from build123d import *

# Parameters (mm, degrees)
F1_DEPTH = 1220
F2_T     = -4


with BuildPart() as f1:
    # F0 (on Right) → F1 (new body)
    with BuildSketch(Plane.YZ):
        with BuildLine():
            Line((0, 40), (0, 0))
            Line((0, 0), (100, 0))
            Line((100, 0), (100, 40))
            ThreePointArc((100, 40), (97.071068, 47.071068), (90, 50))
            Line((90, 50), (10, 50))
            ThreePointArc((10, 50), (2.928932, 47.071068), (0, 40))
        make_face()
    extrude(amount=F1_DEPTH)

    # F2
    f2_openings = [f1.faces().sort_by_distance(p)[0] for p in [
        (610, 50, 0),
        (1220, 50, 24.80288),
        (0, 50, 24.80288),
    ]]
    offset(amount=F2_T, openings=f2_openings)


solid = f1.part
Design review of the part built by this model. Coordinates are the model's own, in mm. A direction names the side the tool comes from. Give positions to 0.01 mm unless a question says otherwise; leave off trailing zeros. Write each loop counter-clockwise with the first axis right and the second up, starting at its lowest first coordinate (ties: lowest second). Pieces come first, ordered by that corner, then holes. Notation, with made-up numbers: M -36,88 L -9,88 A17 cw -9,119 Z; hole C 60.25,41.5 d4. An arc over 180 degrees is marked long. Return JSON: item names as keys, results as strings. Group by question number.
Item 1: Tool access review of faces 4 (the flat face through (601, 51, 46)), 5 (the flat face through (601, 100, 20)): name each direction out of +Z, -Z, +X, -X, +Y, -Y from which nothing blocks a thin tool from reaching the whole face with its end or side.
Item 2: Wall thickness on line 1 along Y through (x, z) = (276, 8); line 2 along Z through (x, y) = (277, 67); line 3 along Z through (x, y) = (221.5, 8): over which ranges is each line inside the solid? List them lowest first.
Item 3: Take a section at C-C (y = 77.5). Give the boundary of the cut face in (x, z), plus the area to 3 significant figures.
Item 4: Take a section at A-A (z = 17). Give the boundary of the cut face in (x, y).
Item 5: Clearance check with a flat-ended pin moving along its axis: pin 1 Ø2 at (x, y) = (367.5, 22.5) entering from -Z. State where the tip first meets the part, or that it passes through.
Item 6: The part is to be moulded in two halves that separate along Y. For faces 1 (the flat face through (601, 0, 20)), 2 (the flat face through (601, 4, 20)), 3 (the flat face through (1220, 50, 47)), say which applies: pulls with the +Y half, pulls with the -Y half, needs draft (parallel to the pull), parting line crosses it, or undercut.
Item 7: Take a section at B-B (x = 614.5). Give the boundary of the cut face in (y, z), plus the area to 3 significant figures.
Return value:
{
 "1": {"face 4": "-Z, +X, -X", "face 5": "+Z, -Z, +X, -X, +Y"},
 "2": {"line 1": "y = 0 to 4, 96 to 100", "line 2": "z = 46 to 50", "line 3": "z = 45.66 to 49.8"},
 "3": {"outline": "M 0,46 L 1220,46 L 1220,50 L 0,50 Z", "area": "4,880 mm2"},
 "4": {"outline": "M 0,0 L 1220,0 L 1220,4 L 0,4 Z; M 0,96 L 1220,96 L 1220,100 L 0,100 Z"},
 "5": {"pin 1": "stops at z = 46"},
 "6": {"face 1": "pulls with the -Y half", "face 2": "undercut", "face 3": "needs draft"},
 "7": {"outline": "M 0,0 L 4,0 L 4,40 A6 cw 10,46 L 90,46 A6 cw 96,40 L 96,0 L 100,0 L 100,40 A10 ccw 90,50 L 10,50 A10 ccw 0,40 Z", "area": "741 mm2"}
}
